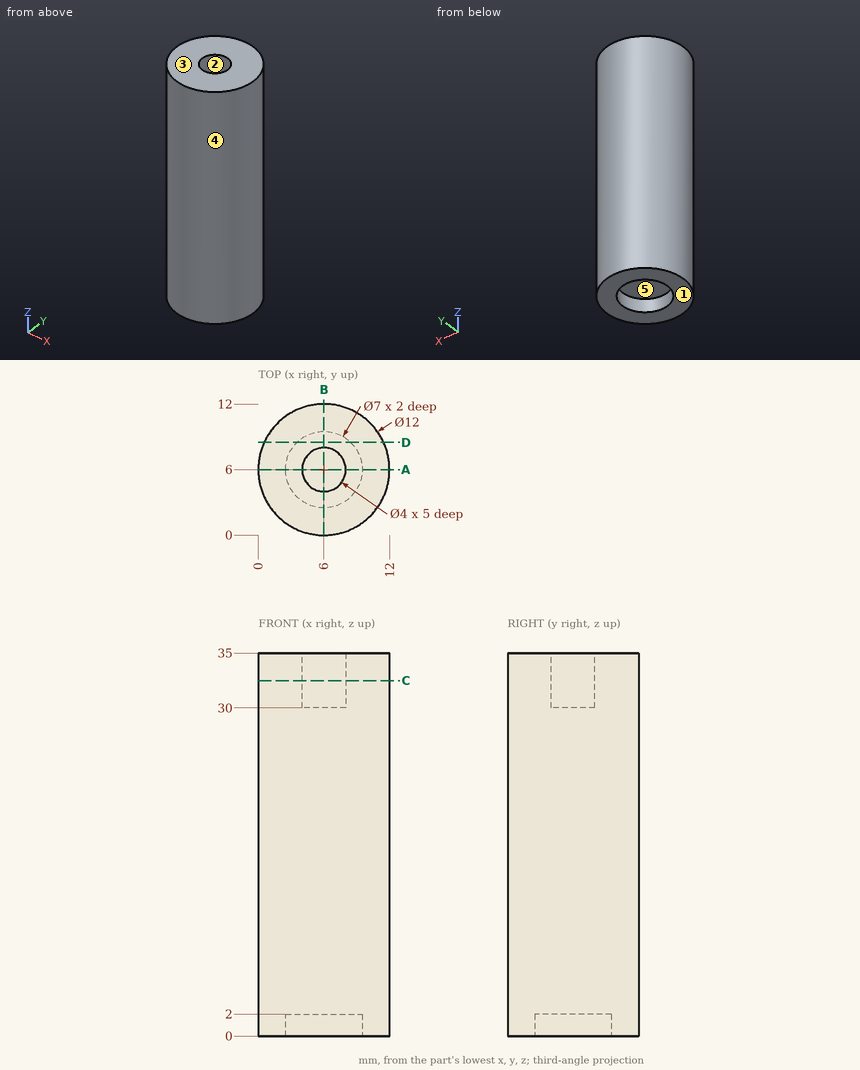
Here's the drawing with two shaded views (mm, measured from the low corner). I have some questions. A direction names the side the tool comes from. Coordinates: 2 decimals unless noted, no trailing zeros. Order: outer loops, then holes, each group sorted by start corner. A loop starts at its lowest first (then second) coordinate and runs counter-clockwise, first axis right, second up. Notation, with made-up numbers: (8, 56.5) - (59, 56.5) arc R18 ccw to (59, 87.5) - close; hole circle Ø5 at (69.5, 31.5). An arc over 180 degrees is marked (long way). Answer in a Markdown table with one row per item. Add a question column.
(1) If we section it at A-A, the plane y = 6: Please give me the cut outline in (x, z).
(2) On a 3-axis mill with a long thin cutter (end or side, diameter ignored), from which of +Z, -Z, +X, -X, +Y, -Y can I reach the whole of each face in a straight line? I mean the marked faces 1 and 2. Say none if no direction works.
(3) Will these pins go through, and if not, where does the flat tip stop? pin 1 (4 mm diameter, centred on y = 8.5, z = 12, fed in from -X); pin 2 (4 mm diameter, centred on x = 6, y = 6, fed in from -Z); pin 3 (1.5 mm diameter, centred on x = 1.5, z = 26.5, fed in from +Y).
(4) If we section it at D-D, the plane y = 8.5: Please give me the cut outline in (x, z), then the cut area to 3 significant figures.
(5) I need wall thicknesses on L1, parallel to Y at x = 6, z = 32; L2, parallel to Y at x = 6, z = 0.85; L3, parallel to Y at x = 5.75, z = 21.5. Which ranges of each line are inside material? Lowest first, please.
(6) If we section it at C-C, the plane z = 32.5: Please give me the cut outline in (x, y), then the cut area to 3 significant figures.
(7) If we mould it in two halves opening along X, with no side actions, what happens to the marked faces 3, 4 and 5? For each: released by +X, released by -X, zero draft, split by the parting line, or undercut.
Results are:
| question | item | result |
|---|---|---|
| 1 | outline | (0, 0) - (2.5, 0) - (2.5, 2) - (9.5, 2) - (9.5, 0) - (12, 0) - (12, 35) - (8, 35) - (8, 30) - (4, 30) - (4, 35) - (0, 35) - close |
| 2 | face 1 | -Z, +X, -X, +Y, -Y |
| 2 | face 2 | +Z |
| 3 | pin 1 | stops at x = 0.02 |
| 3 | pin 2 | stops at z = 2 |
| 3 | pin 3 | stops at y = 10.68 |
| 4 | outline | (0.55, 0) - (3.55, 0) - (3.55, 2) - (8.45, 2) - (8.45, 0) - (11.45, 0) - (11.45, 35) - (0.55, 35) - close |
| 4 | area | 372 mm2 |
| 5 | L1 | y = 0 to 4, 8 to 12 |
| 5 | L2 | y = 0 to 2.5, 9.5 to 12 |
| 5 | L3 | y = 0.01 to 11.99 |
| 6 | outline | circle Ø12 at (6, 6); hole circle Ø4 at (6, 6) |
| 6 | area | 101 mm2 |
| 7 | face 3 | zero draft |
| 7 | face 4 | split by the parting line |
| 7 | face 5 | undercut |
